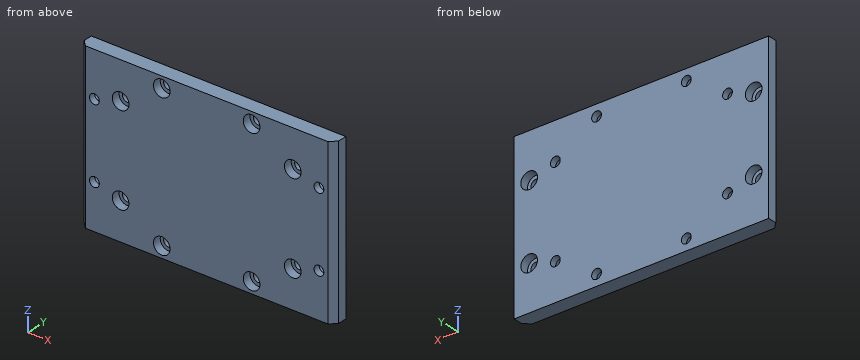
```python
from build123d import *

# Parameters (mm, degrees)
SKETCH2_W                                      = 55
SKETCH2_H                                      = 55
BOSS_EXTRUDE1_DEPTH                            = 5
SKETCH6_W                                      = 15
SKETCH6_H                                      = 55
BOSS_EXTRUDE2_DEPTH                            = 5
CBORE_FOR_4_SOCKET_HEAD_CAP_SCREW2_D           = 3.2639
CBORE_FOR_4_SOCKET_HEAD_CAP_SCREW2_CBORE_D     = 5.55752
CBORE_FOR_4_SOCKET_HEAD_CAP_SCREW2_CBORE_DEPTH = 2.8448
CBORE_FOR_4_SOCKET_HEAD_CAP_SCREW3_D           = 3.2639
CBORE_FOR_4_SOCKET_HEAD_CAP_SCREW3_CBORE_D     = 5.55752
CBORE_FOR_4_SOCKET_HEAD_CAP_SCREW3_CBORE_DEPTH = 2.8448
CHAMFER1_SIZE                                  = 2


with BuildPart() as part:
    # Sketch2 → Boss-Extrude1 (new body)
    with BuildSketch(Plane(origin=(0, 0, 0), x_dir=(1, 0, 0), z_dir=(0, 1, 0))):
        Rectangle(SKETCH2_W, SKETCH2_H)
    extrude(amount=BOSS_EXTRUDE1_DEPTH)

    # Sketch6 → Boss-Extrude2 (add)
    with BuildSketch(Plane.XZ):
        with Locations((-35, 0)):
            Rectangle(SKETCH6_W, SKETCH6_H)
        with Locations((35, 0)):
            Rectangle(SKETCH6_W, SKETCH6_H)
    extrude(amount=-BOSS_EXTRUDE2_DEPTH)

    # CBORE for #4 Socket Head Cap Screw2 (through all)
    with Locations(Plane(origin=(0, 5, 0), x_dir=(1, 0, 0), z_dir=(0, 1, 0))):
        with Locations((-37.5, 12.5), (-37.5, -12.5), (37.5, -12.5), (37.5, 12.5)):
            CounterBoreHole(CBORE_FOR_4_SOCKET_HEAD_CAP_SCREW2_D / 2, CBORE_FOR_4_SOCKET_HEAD_CAP_SCREW2_CBORE_D / 2, CBORE_FOR_4_SOCKET_HEAD_CAP_SCREW2_CBORE_DEPTH)

    # CBORE for #4 Socket Head Cap Screw3 (through all)
    with Locations(Plane(origin=(0, 0, 0), x_dir=(-1, 0, 0), z_dir=(0, -1, 0))):
        with Locations((-28.75, 15), (-15, 23.75), (-28.75, -15), (-15, -23.75), (15, -23.75), (28.75, -15), (28.75, 15), (15, 23.75)):
            CounterBoreHole(CBORE_FOR_4_SOCKET_HEAD_CAP_SCREW3_D / 2, CBORE_FOR_4_SOCKET_HEAD_CAP_SCREW3_CBORE_D / 2, CBORE_FOR_4_SOCKET_HEAD_CAP_SCREW3_CBORE_DEPTH)

    # Chamfer1
    chamfer1_edges = [part.edges().sort_by_distance(p)[0] for p in [
        (-42.5, 0, 0),
        (42.5, 0, 0),
    ]]
    chamfer(chamfer1_edges, length=CHAMFER1_SIZE)


solid = part.part
```
Model file for the job. Use its own axes, mm. Coordinates: 2 decimals unless noted, no trailing zeros. Write each loop counter-clockwise with the first axis right and the second up, starting at its lowest first coordinate (ties: lowest second). Pieces come first, ordered by that corner, then holes. Notation, with made-up numbers: (71.5, 1) - (108.5, 1) arc R34 ccw to (108.5, 39) - close; hole circle Ø3 at (31, 3). An arc over 180 degrees is marked (long way). One line per item, written item: value. Start each with the question number.
1. Probe line 1 (Z direction, x = -15, y = 3.6); line 2 (Z direction, x = 37.5, y = 1.45); line 3 (X direction, y = 4.1, z = 23.75). List the from-to ranges inside material, lowest first. Write a range as from..to.
2. Slice it at B-B (y = 0.8). Count the separate pieces of the cut face and the enclosed holes in it, plus the area to 3 significant figures.
3. Flat gauge pins, fed straight in: pin 1 (6 mm diameter, centred on x = -37.5, z = 12.5, fed in from +Y); pin 2 (3 mm diameter, centred on x = -37.5, z = 12.5, fed in from -Y); pin 3 (4 mm diameter, centred on x = -28.75, z = -15, fed in from -Y). Where does each tip first touch, or does it go through?
4. Slice it at A-A (x = 28.75). Write the cut outline in (y, z), plus the area to 3 significant figures.
Answers below:
1. line 1: z = -27.5..-25.38, -22.12..22.12, 25.38..27.5
1. line 2: z = -27.5..-14.13, -10.87..10.87, 14.13..27.5
1. line 3: x = -42.5..-16.63, -13.37..13.37, 16.63..42.5
2. separate pieces: 1
2. enclosed holes: 12
2. area: 4,320 mm^2
3. pin 1: stops at y = 5
3. pin 2: passes through
3. pin 3: stops at y = 2.84
4. outline: (0, -27.5) - (5, -27.5) - (5, -16.63) - (2.84, -16.63) - (2.84, -17.78) - (0, -17.78) - close; (0, -12.22) - (2.84, -12.22) - (2.84, -13.37) - (5, -13.37) - (5, 13.37) - (2.84, 13.37) - (2.84, 12.22) - (0, 12.22) - close; (0, 17.78) - (2.84, 17.78) - (2.84, 16.63) - (5, 16.63) - (5, 27.5) - (0, 27.5) - close
4. area: 229 mm^2
